Read the model definition and answer for the solid it produces. Units are mm, in the model's axes. Face numbers are marked on the shaded views. A direction names the side the tool comes from. Give positions to 0.01 mm unless a question says otherwise; leave off trailing zeros. Write each loop counter-clockwise with the first axis right and the second up, starting at its lowest first coordinate (ties: lowest second). Pieces come first, ordered by that corner, then holes.
```python
from build123d import *


with BuildPart() as part:
    # Sketch1 → Revolve-Thin7 (revolve)
    with BuildSketch(Plane.XY, mode=Mode.PRIVATE) as revolve_thin7_sk:
        Polygon((5, 0), (7, 0), (7, 8), (9, 10.5), (9, 13), (4, 13), align=None)
        Polygon((5.000092603, 0.0001), (6.9999, 0.0001), (6.9999, 8.000035078), (8.9999, 10.500035078), (8.9999, 12.9999), (4.000107988, 12.9999), align=None, mode=Mode.SUBTRACT)
    revolve(revolve_thin7_sk.sketch.rotate(Axis((0, 0, 0), (0, 1, 0)), 270), axis=Axis((0, 0, 0), (0, 1, 0)))


solid = part.part
```
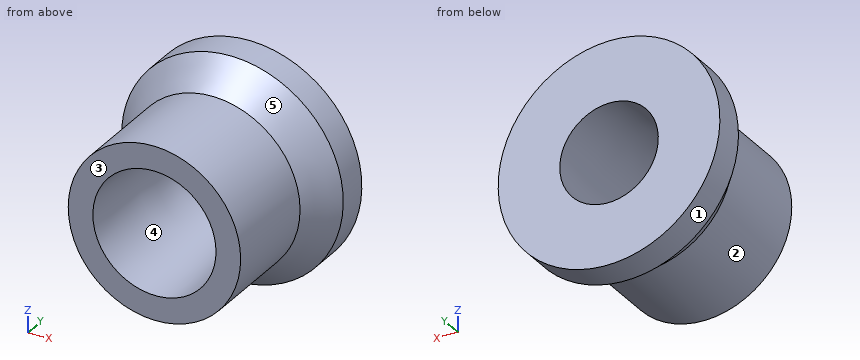
Item 1: Section A-A (x = 0) is taken. Write down the section's boundary in (y, z).
Result set:
outline: (0, -7) - (8, -7) - (10.5, -9) - (13, -9) - (13, -4) - (0, -5) - close; (0, 5) - (13, 4) - (13, 9) - (10.5, 9) - (8, 7) - (0, 7) - close; hole (0, -7) - (8, -7) - (10.5, -9) - (13, -9) - (13, -4) - (0, -5) - close; hole (0, 5) - (13, 4) - (13, 9) - (10.5, 9) - (8, 7) - (0, 7) - close
Item 2: Section B-B (z = 0) is taken. Write down the section's boundary in (x, y), and give its area (3 significant figures).
Result set:
outline: (-9, 10.5) - (-7, 8) - (-7, 0) - (-5, 0) - (-4, 13) - (-9, 13) - close; (4, 13) - (5, 0) - (7, 0) - (7, 8) - (9, 10.5) - (9, 13) - close; hole (-9, 10.5) - (-7, 8) - (-7, 0) - (-5, 0) - (-4, 13) - (-9, 13) - close; hole (4, 13) - (5, 0) - (7, 0) - (7, 8) - (9, 10.5) - (9, 13) - close
area: 0.00675 mm2
Item 3: Section C-C (y = 11) is taken. Write down the section's boundary in (x, z), and give its area (3 significant figures).
Result set:
outline: circle Ø18 at (0, 0); circle Ø8.31 at (0, 0); hole circle Ø18 at (0, 0); hole circle Ø8.31 at (0, 0)
area: 0.00827 mm2
Item 4: Section D-D (y = 8.75) is taken. Write down the section's boundary in (x, z).
Result set:
outline: circle Ø15.2 at (0, 0); circle Ø8.65 at (0, 0); hole circle Ø15.2 at (0, 0); hole circle Ø8.65 at (0, 0)
Item 5: Determine the mould class of the marked faces 3, 4 and 5 for opening direction Z: pulls with the +Z half, pulls with the -Z half, needs draft (parallel to the pull), parting line crosses it, or undercut.
Result set:
face 3: needs draft
face 4: undercut
face 5: parting line crosses it
Item 6: Each of these flat-tipped pins is pushed along its axis until it touches: pin 1 Ø3 at (y, z) = (8, -7) entering from +X; pin 2 Ø4 at (y, z) = (5, 3.5) entering from +X; pin 3 Ø4 at (x, y) = (6, 9.5) entering from -Z. Where does it stop, or does it pass through?
Result set:
pin 1: stops at x = 5.13
pin 2: stops at x = 6.84
pin 3: stops at z = -7.92
Item 7: Which of the six approach directions +Z, -Z, +X, -X, +Y, -Y give full straight-line access (tool end or side, diameter ignored) to the marked faces 1 and 2?
Result set:
face 1: +Y, -Y
face 2: -Y
